Could you check a few things on this model? Use its own coordinates, in mm. A direction names the side the tool comes from. Give positions to 0.01 mm unless a question says otherwise; leave off trailing zeros. Loops run counter-clockwise (first coordinate to the right, second up) from the corner with the lowest first, then second, coordinate; pieces in that order, holes last. Notation, with made-up numbers: M -14,16 L 24,16 A29 ccw 24,39 Z; hole C -24.75,23.25 d2. An arc over 180 degrees is marked long. Use a Markdown table: item, result. Add a question column.
1) Suppose I cut it at B-B on z = 6.5. List the corners of the cut face in (x, y) for me.
2) Will these pins go through, and if not, where does the flat tip stop? pin 1 Ø1.5 at (y, z) = (1.5, -5) entering from +X; pin 2 Ø1.5 at (x, z) = (-29.5, -2) entering from +Y; pin 3 Ø4.5 at (x, y) = (-24, 9.5) entering from -Z.
3) Which directions (+Z, -Z, +X, -X, +Y, -Y) give clear straight access to the entire face, cutting with the end or side of a thin tool? Please do faces 1 (the flat face through (-31.3, 3, -2)), 2 (the flat face through (-34, 8, 10)), 3 (the cylindrical face through (-17.56, 6.08, 1.48)), 4 (the flat face through (-28.3, 3, -4)).
4) We'd pull the mould along X, two halves only. Please class faces 5 (the flat face through (-36, 5, 9.3)), 6 (the flat face through (-24.3, 10, 8)), 7 (the flat face through (-40.4, 12, 7)): +X half, -X half, draft (parallel to the pull), parting line (faces both ways), or undercut.
5) Suppose I cut it at C-C on y = 10.25. List the corners of the cut face in (x, z) for me, and give its area (3 significant figures).
6) If I drill on line 1 along Z through (x, y) = (-36.5, 12.75); line 2 along X through (y, z) = (7.35, 6.5); line 3 along X through (y, z) = (1.25, 0.75), over which ranges is the centre line in solid material (lowest first)? Write a range as [from, to].
7) Suppose I cut it at A-A on y = 7.5. List the corners of the cut face in (x, z) for me, and give its area (3 significant figures).
8) Suppose I cut it at D-D on z = 1. List the corners of the cut face in (x, y) for me.
```python
from build123d import *

# Parameters (mm, degrees)
CROQUIS1_R              = 1.6
SALIENTE_EXTRUIR1_DEPTH = 3
CROQUIS2_W              = 19
CROQUIS2_H              = 10
SALIENTE_EXTRUIR2_DEPTH = 10
CROQUIS3_W              = 13.2
CROQUIS3_H              = 7.2
CORTAR_EXTRUIR1_DEPTH   = 7
CROQUIS4_R              = 3.2
CORTAR_EXTRUIR2_DEPTH   = 3
CROQUIS5_W              = 10
CROQUIS5_H              = 5
SALIENTE_EXTRUIR3_DEPTH = 3


with BuildPart() as part:
    # Croquis1 → Saliente-Extruir1 (new body)
    with BuildSketch(Plane.XY):
        Polygon((-13.299831285, 0), (-28.299831285, 0), (-28.299831285, 5), (-43.299831285, 5), (-43.299831285, 15), (-13.299831285, 15), align=None)
        with Locations((-18.299831285, 7.5)):
            Circle(CROQUIS1_R, mode=Mode.SUBTRACT)
    extrude(amount=SALIENTE_EXTRUIR1_DEPTH)

    # Croquis2 → Saliente-Extruir2 (add)
    with BuildSketch(Plane.XY.offset(3)):
        with Locations((-33.799831285, 10)):
            Rectangle(CROQUIS2_W, CROQUIS2_H)
    extrude(amount=SALIENTE_EXTRUIR2_DEPTH)

    # Croquis3 → Cortar-Extruir1 (cut)
    with BuildSketch(Plane(origin=(0, 15, 0), x_dir=(1, 0, 0), z_dir=(0, 1, 0))):
        with Locations((-33.799831285, -6.6)):
            Rectangle(CROQUIS3_W, CROQUIS3_H)
    extrude(amount=-CORTAR_EXTRUIR1_DEPTH, mode=Mode.SUBTRACT)

    # Croquis4 → Cortar-Extruir2 (cut)
    with BuildSketch(Plane(origin=(0, 8, 0), x_dir=(1, 0, 0), z_dir=(0, 1, 0))):
        with Locations((-33.799831285, -6.5)):
            Circle(CROQUIS4_R)
    extrude(amount=-CORTAR_EXTRUIR2_DEPTH, mode=Mode.SUBTRACT)

    # Croquis5 → Saliente-Extruir3 (add)
    with BuildSketch(Plane.ZY.offset(28.299831285)):
        with Locations((-2, 2.5)):
            Rectangle(CROQUIS5_W, CROQUIS5_H)
    extrude(amount=SALIENTE_EXTRUIR3_DEPTH)


solid = part.part
```
Answer block:
| question | item | result |
|---|---|---|
| 1 | outline | M -43.3,5 L -37,5 L -37,8 L -40.4,8 L -40.4,15 L -43.3,15 Z; M -30.6,5 L -24.3,5 L -24.3,15 L -27.2,15 L -27.2,8 L -30.6,8 Z |
| 2 | pin 1 | stops at x = -28.3 |
| 2 | pin 2 | stops at y = 5 |
| 2 | pin 3 | stops at z = 0 |
| 3 | face 1 | +Z, -Z, -X, -Y |
| 3 | face 2 | +Y |
| 3 | face 3 | +Z, -Z |
| 3 | face 4 | -Z, +X, +Y, -Y |
| 4 | face 5 | draft |
| 4 | face 6 | +X half |
| 4 | face 7 | undercut |
| 5 | outline | M -43.3,0 L -13.3,0 L -13.3,3 L -24.3,3 L -24.3,13 L -43.3,13 Z; hole M -40.4,3 L -27.2,3 L -27.2,10.2 L -40.4,10.2 Z |
| 5 | area | 185 mm^2 |
| 6 | line 1 | z = [0, 3], [10.2, 13] |
| 6 | line 2 | x = [-43.3, -37], [-30.6, -24.3] |
| 6 | line 3 | x = [-31.3, -13.3] |
| 7 | outline | M -43.3,0 L -19.9,0 L -19.9,3 L -24.3,3 L -24.3,13 L -43.3,13 Z; M -16.7,0 L -13.3,0 L -13.3,3 L -16.7,3 Z; hole C -33.8,6.5 d6.4 |
| 7 | area | 238 mm^2 |
| 8 | outline | M -43.3,5 L -31.3,5 L -31.3,0 L -13.3,0 L -13.3,15 L -43.3,15 Z; hole C -18.3,7.5 d3.2 |
